Read the model definition and answer for the solid it produces. Units are mm, in the model's axes. A direction names the side the tool comes from. Coordinates: 2 decimals unless noted, no trailing zeros. Loops run counter-clockwise (first coordinate to the right, second up) from the corner with the lowest first, then second, coordinate; pieces in that order, holes last. Notation, with made-up numbers: M 37,85 L 77,85 A21 ccw 77,124 Z; hole C 13.25,4.25 d10. An arc over 180 degrees is marked long. One line per item, written item: value. Start each with the question number.
1. The part is cut by section A-A (z = -64.5). Write down the section's boundary in (x, y).
2. Flat-ended cylindrical pins translate along their axes: pin 1 (3 mm diameter, centred on y = 53, z = -55.5, fed in from -X); pin 2 (3 mm diameter, centred on y = 47, z = -34, fed in from -X); pin 3 (1 mm diameter, centred on x = -26, z = -18, fed in from +Y). Find the tip coordinate at first contact, or state that the pin passes through.
3. The part is cut by section D-D (z = -32.5). Write down the section's boundary in (x, y).
4. For faces 4 (the face through (25.379, 48.794, -65.07)), 5 (the face through (11, -58, -67)), 6 (the face through (-19, 52, 0)), 7 (the face through (25.379, 48.794, -5.07)), determine the directions among +Z, -Z, +X, -X, +Y, -Y from which every point of the face is accessible in a straight line to the end or side of a thin tool.
5. Consider probe 1 along Y at (x, z) = (0, -6.25); probe 2 along Z at (x, y) = (-60.5, 31); probe 3 along Y at (x, z) = (-6.5, -56). Determine where each line is inside the solid, lowest interval first.
6. Determine the mould class of faces 1 (the face through (-63.68, 48.82, -34.51)), 2 (the face through (26.76, 51.46, -63.25)), 3 (the face through (19, 52, -70)) for opening direction Y: +Y half, -Y half, draft (parallel to the pull), parting line (faces both ways), or undercut.
```python
from build123d import *


with BuildPart() as part:
    # 草圖4 → 旋轉1 (revolve)
    with BuildSketch(Plane(origin=(0, 0, 0), x_dir=(0, 0, -1), z_dir=(1, 0, 0)), mode=Mode.PRIVATE) as revolve_1_sk:
        with BuildLine():
            Line((0, 55), (10, 55))
            ThreePointArc((10, 55), (12.745508857, 54.295513936), (15.502645054, 53.638003865))
            Line((15.502645054, 53.638003865), (15.502645054, 56.7174692))
            ThreePointArc((15.502645054, 56.7174692), (12.942937744, 57.338097036), (10.393591772, 58))
            Line((10.393591772, 58), (3, 58))
            Line((3, 58), (3, 77.239932534))
            Line((3, 77.239932534), (67, 77.239932534))
            Line((67, 77.239932534), (67, 58))
            Line((67, 58), (59.606408228, 58))
            ThreePointArc((59.606408228, 58), (57.057062256, 57.338097036), (54.497354946, 56.7174692))
            Line((54.497354946, 56.7174692), (54.497354946, 53.638003865))
            ThreePointArc((54.497354946, 53.638003865), (57.254491143, 54.295513936), (60, 55))
            Line((60, 55), (70, 55))
            Line((70, 55), (70, 80.239932534))
            Line((70, 80.239932534), (0, 80.239932534))
            Line((0, 80.239932534), (0, 55))
        make_face()
    revolve(revolve_1_sk.sketch.rotate(Axis((0, 0, 0), (0, 0, -1)), 90), axis=Axis((0, 0, 0), (0, 0, -1)))


solid = part.part
```
Answer block:
1. outline: C 0,0 d160.48; C 0,0 d116; hole C 0,0 d154.48; hole C 0,0 d110
2. pin 1: stops at x = -61.53
2. pin 2: stops at x = -66.09
2. pin 3: stops at y = 76.08
3. outline: C 0,0 d160.48; hole C 0,0 d154.48
4. face 4: -Z
4. face 5: none
4. face 6: +Z, +X, -X, +Y, -Y
4. face 7: +Z
5. probe 1: y = -80.24 to -77.24, -58 to -55, 55 to 58, 77.24 to 80.24
5. probe 2: z = -70 to -67, -3 to 0
5. probe 3: y = -79.98 to -76.97, -56.71 to -53.6, 53.6 to 56.71, 76.97 to 79.98
6. face 1: parting line
6. face 2: undercut
6. face 3: draft
